Here's the drawing with two shaded views (mm, measured from the low corner). I have some questions. A direction names the side the tool comes from. Coordinates: 2 decimals unless noted, no trailing zeros. Write each loop counter-clockwise with the first axis right and the second up, starting at its lowest first coordinate (ties: lowest second). Pieces come first, ordered by that corner, then holes.
Item 1: If we section it at C-C (y = 10): Please give me the cut outline in (x, z).
Item 2: If we section it at B-B (y = 2.5): Count the separate pieces of the cut face and the enclosed holes in it.
Item 3: For the marked faces 1 and 2, which set-ups out of +Z, -Z, +X, -X, +Y, -Y let a thin tool reach every point of the face, with its end or its side?
Item 4: If I drill on line 1 (Y direction, x = 6.75, z = 0.75); line 2 (X direction, y = 17.25, z = 0.4); line 3 (Z direction, x = 26.5, y = 2), over which ranges is the centre line in solid material (lowest first)?
Item 5: If we section it at A-A (x = 21.75): Please give me the cut outline in (y, z), then the cut area to 3 significant figures.
Item 6: I'm going to push flat-ended pins straight in: pin 1 Ø1.8 at (x, y) = (21.75, 24.85) entering from -Z; pin 2 Ø0.8 at (x, z) = (10, 0.5) entering from -Y; pin 3 Ø2 at (x, y) = (24.5, 2.5) entering from +Z. Where does each tip first touch, or does it pass through?
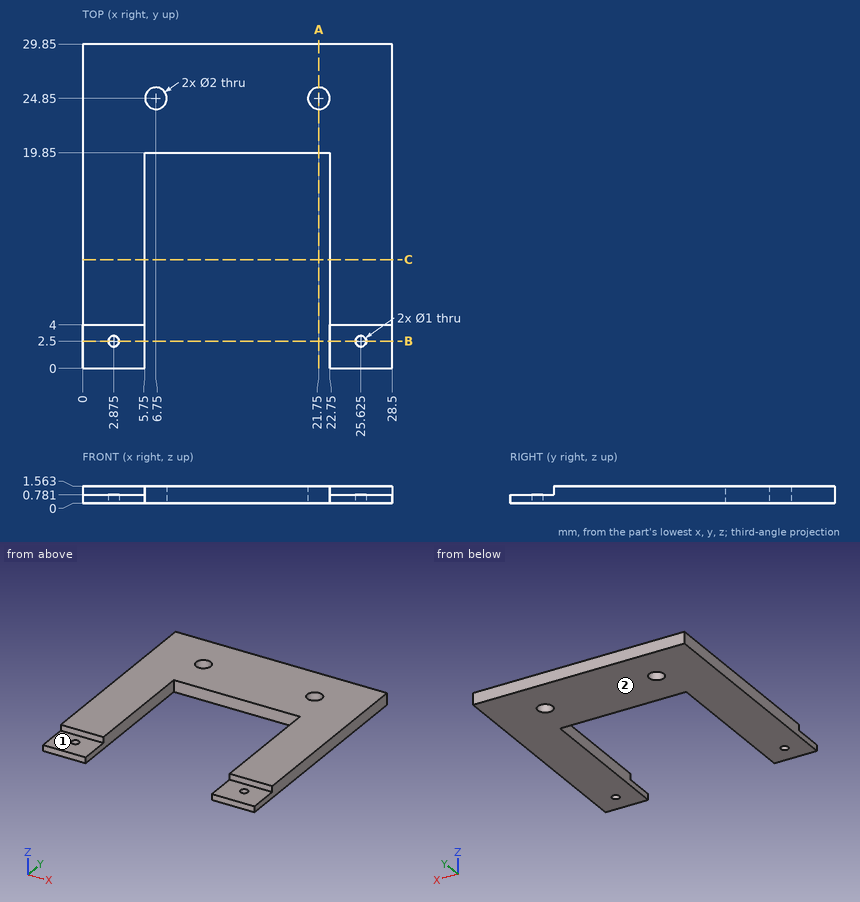
Answer list:
1. outline: (0, 0) - (5.75, 0) - (5.75, 1.56) - (0, 1.56) - close; (22.75, 0) - (28.5, 0) - (28.5, 1.56) - (22.75, 1.56) - close
2. separate pieces: 4
2. enclosed holes: 0
3. face 1: +Z, +X, -X, -Y
3. face 2: -Z, +X, -X, +Y, -Y
4. line 1: y = 19.85 to 23.85, 25.85 to 29.85
4. line 2: x = 0 to 5.75, 22.75 to 28.5
4. line 3: z = 0 to 0.78
5. outline: (19.85, 0) - (23.85, 0) - (23.85, 1.56) - (19.85, 1.56) - close; (25.85, 0) - (29.85, 0) - (29.85, 1.56) - (25.85, 1.56) - close
5. area: 12.5 mm2
6. pin 1: passes through
6. pin 2: stops at y = 19.85
6. pin 3: stops at z = 0.78
